The drawing under review shows one solid part. Ordinate dimensions are in mm from its lowest x, y, z. A direction names the side the tool comes from. Coordinates: 2 decimals unless noted, no trailing zeros. Write each loop counter-clockwise with the first axis right and the second up, starting at its lowest first coordinate (ties: lowest second). Pieces come first, ordered by that corner, then holes.
1) For the marked faces 5 and 6, list the 3-axis set-ups (+Z, -Z, +X, -X, +Y, -Y) from which the entire face can be reached by the end or side of a thin tool; tool diameter is ignored.
2) We need section C-C on y = 18. Write out the cut boundary in (x, z), then the cut area to 3 significant figures.
3) Mouldability with a two-part tool opening along X and no side actions: class the marked faces 1, 2, 3 and 4 as pulls with the +X half, pulls with the -X half, needs draft (parallel to the pull), parting line crosses it, or undercut.
4) We need section B-B on z = 15. Write out the cut boundary in (x, y), then the cut area to 3 significant figures.
5) To check wall thickness, follow line 1 along Z through (x, y) = (28.7, 10); line 2 along X through (y, z) = (9.25, 12.5); line 3 along Z through (x, y) = (42, 23.5). State the ranges of each line that lie inside material, in increasing order.
6) Insertion check: P1, Ø10, axis at x = 19.5, y = 6.5, coming from the +Z side; P2, Ø1.5, axis at x = 22.5, z = 2.5, coming from the -Y side; P3, Ø10, axis at y = 12.5, z = 9.5, coming from the +X side. Each pin has a flat end and moves straight along its axis. Give the tip position at first contact, or say it passes through.
7) We need section D-D on x = 16. Write out the cut boundary in (y, z).
8) We need section A-A on y = 10. Write out the cut boundary in (x, z), then the cut area to 3 significant figures.
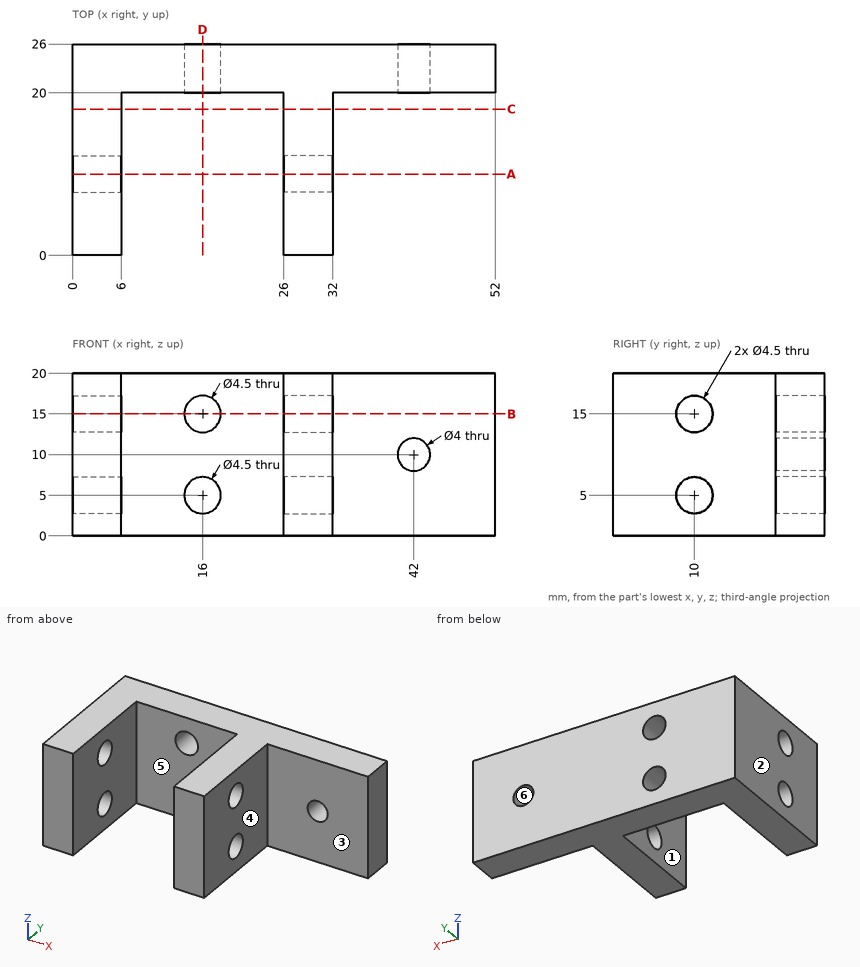
Result:
1. face 5: +Z, -Z, -Y
1. face 6: +Y, -Y
2. outline: (0, 0) - (6, 0) - (6, 20) - (0, 20) - close; (26, 0) - (32, 0) - (32, 20) - (26, 20) - close
2. area: 240 mm2
3. face 1: undercut
3. face 2: pulls with the -X half
3. face 3: needs draft
3. face 4: pulls with the +X half
4. outline: (0, 0) - (6, 0) - (6, 7.75) - (0, 7.75) - close; (0, 12.25) - (6, 12.25) - (6, 20) - (13.75, 20) - (13.75, 26) - (0, 26) - close; (18.25, 20) - (26, 20) - (26, 12.25) - (32, 12.25) - (32, 20) - (52, 20) - (52, 26) - (18.25, 26) - close; (26, 0) - (32, 0) - (32, 7.75) - (26, 7.75) - close
4. area: 471 mm2
5. line 1: z = 0 to 2.75, 7.25 to 12.75, 17.25 to 20
5. line 2: x = 0 to 6, 26 to 32
5. line 3: z = 0 to 8, 12 to 20
6. P1: passes through
6. P2: stops at y = 20
6. P3: stops at x = 32
7. outline: (20, 0) - (26, 0) - (26, 2.75) - (20, 2.75) - close; (20, 7.25) - (26, 7.25) - (26, 12.75) - (20, 12.75) - close; (20, 17.25) - (26, 17.25) - (26, 20) - (20, 20) - close
8. outline: (0, 0) - (6, 0) - (6, 2.75) - (0, 2.75) - close; (0, 7.25) - (6, 7.25) - (6, 12.75) - (0, 12.75) - close; (0, 17.25) - (6, 17.25) - (6, 20) - (0, 20) - close; (26, 0) - (32, 0) - (32, 2.75) - (26, 2.75) - close; (26, 7.25) - (32, 7.25) - (32, 12.75) - (26, 12.75) - close; (26, 17.25) - (32, 17.25) - (32, 20) - (26, 20) - close
8. area: 132 mm2
